The listing builds one solid part. Answer for the finished solid, in the listing's coordinates (mm). A direction names the side the tool comes from. Give positions to 0.01 mm unless a question says otherwise; leave off trailing zeros. Loops run counter-clockwise (first coordinate to the right, second up) from the corner with the lowest first, then second, coordinate; pieces in that order, holes last. Notation, with made-up numbers: (12.25, -32) - (29.25, -32) arc R29 cw to (29.25, -3) - close; hole circle Ø1 at (53.5, -16). An arc over 180 degrees is marked (long way). Write each question's results on one line, items separated by ' | '.
from build123d import *

# Parameters (mm, degrees)
F0_W      = 609.6
F0_H      = 609.6
F0_W_2    = 571.5
F0_H_2    = 571.5
F1_DEPTH  = 381
F3_DEPTH  = 25.4
F5_DEPTH  = 25.4
F6_R      = 5.08
F7_W      = 812.8
F7_H      = 711.2
F8_DEPTH  = 19.05
F9_W      = 812.8
F9_H      = 711.2
F9_W_2    = 774.7
F9_H_2    = 673.1
F10_DEPTH = 101.6
F11_W     = 101.6
F11_H     = 50.8
F12_DEPTH = 711.201
F13_W     = 101.6
F13_H     = 50.8
F14_DEPTH = 812.801


with BuildPart() as f1:
    # F0 (on Top) → F1 (new body, symmetric)
    with BuildSketch(Plane.XY):
        Rectangle(F0_W, F0_H)
        Rectangle(F0_W_2, F0_H_2, mode=Mode.SUBTRACT)
    extrude(amount=F1_DEPTH, both=True)

    # F2 (on face) → F3 (cut)
    with BuildSketch(Plane.XZ.offset(304.8)):
        with BuildLine():
            Line((-228.6, -76.2), (-228.6, -381))
            Line((-228.6, -381), (228.6, -381))
            Line((228.6, -381), (228.6, -76.2))
            ThreePointArc((228.6, -76.2), (0, 152.4), (-228.6, -76.2))
        make_face()
    extrude(amount=-F3_DEPTH, mode=Mode.SUBTRACT)

    # F4 (on face) → F5 (cut)
    with BuildSketch(Plane.YZ.offset(304.8)):
        with BuildLine():
            Line((-228.6, -76.2), (-228.6, -381))
            Line((-228.6, -381), (228.6, -381))
            Line((228.6, -381), (228.6, -76.2))
            ThreePointArc((228.6, -76.2), (0, 152.4), (-228.6, -76.2))
        make_face()
    extrude(amount=-F5_DEPTH, mode=Mode.SUBTRACT)

    # F6
    f6_edges = [f1.edges().sort_by_distance(p)[0] for p in [
        (-228.6, -304.8, -228.6),
        (-228.6, -295.275, -381),
        (-228.6, -285.75, -228.6),
        (-228.6, -295.275, -76.2),
        (0, -304.8, 152.4),
        (0, -285.75, 152.4),
        (228.6, -295.275, -76.2),
        (228.6, -304.8, -228.6),
        (228.6, -285.75, -228.6),
        (228.6, -295.275, -381),
    ]]
    fillet(f6_edges, radius=F6_R)

    # F7 (on face) → F8 (join)
    with BuildSketch(Plane.XY.offset(381)):
        with Locations((0, -50.8)):
            Rectangle(F7_W, F7_H)
    extrude(amount=F8_DEPTH)

    # F9 (on face) → F10 (join)
    with BuildSketch(Plane.XY.offset(400.05)):
        with Locations((0, -50.8)):
            Rectangle(F9_W, F9_H)
        with Locations((0, -50.8)):
            Rectangle(F9_W_2, F9_H_2, mode=Mode.SUBTRACT)
    extrude(amount=F10_DEPTH)

    # F11 (on face) → F12 (cut, through all)
    with BuildSketch(Plane.XZ.offset(406.4)):
        with Locations((-228.6, 476.25)):
            Rectangle(F11_W, F11_H)
        with Locations((-2.54, 476.25)):
            Rectangle(F11_W, F11_H)
        with Locations((223.52, 476.25)):
            Rectangle(F11_W, F11_H)
    extrude(amount=-F12_DEPTH, mode=Mode.SUBTRACT)

    # F13 (on face) → F14 (cut, through all)
    with BuildSketch(Plane(origin=(-406.4, 0, 0), x_dir=(0, -1, 0), z_dir=(-1, 0, 0))):
        with Locations((-152.4, 476.25)):
            Rectangle(F13_W, F13_H)
        with Locations((53.34, 476.25)):
            Rectangle(F13_W, F13_H)
        with Locations((259.08, 476.25)):
            Rectangle(F13_W, F13_H)
    extrude(amount=-F14_DEPTH, mode=Mode.SUBTRACT)


solid = f1.part
Item 1: Flat-ended cylindrical pins translate along their axes: P1, Ø3, axis at x = 217.5, y = 71.5, coming from the -Z side; P2, Ø8, axis at y = -66, z = 156, coming from the -X side; P3, Ø12, axis at x = -62, z = 321, coming from the -Y side. Find the tip coordinate at first contact, or state that the pin passes through.
Values found:
P1: stops at z = 381 | P2: stops at x = -304.8 | P3: stops at y = -304.8
Item 2: For a pull along Y with two mould halves and no side action, classify faces 1 (the face through (5.027, -295.337, 152.345)), 2 (the face through (-4, -285.75, 175)), 3 (the face through (-6, 304.8, 54)) as released by +Y, released by -Y, zero draft, split by the parting line, or undercut.
Values found:
face 1: zero draft | face 2: undercut | face 3: released by +Y
Item 3: Find the intervals of material crossed by line 1 along Y through (x, z) = (23, 429); line 2 along Y through (x, z) = (297, -116); line 3 along Z through (x, y) = (277.5, -141), in increasing order. Write a range as [from, to].
Values found:
line 1: y = [-406.4, -387.35], [285.75, 304.8] | line 2: y = [-304.8, -228.6], [228.6, 304.8] | line 3: z = [381, 400.05]
Item 4: A cutting plane is placed at B-B, the plane x = -258. Determine the outline of the cut face in (y, z).
Values found:
outline: (-406.4, 381) - (-304.8, 381) - (-304.8, -381) - (-285.75, -381) - (-285.75, 381) - (285.75, 381) - (285.75, -381) - (304.8, -381) - (304.8, 450.85) - (285.75, 450.85) - (285.75, 400.05) - (-387.35, 400.05) - (-387.35, 450.85) - (-406.4, 450.85) - close
Item 5: A cutting plane is placed at A-A, the plane z = -269.5. Determine the outline of the cut face in (x, y).
Values found:
outline: (-304.8, -304.8) - (-233.68, -304.8) arc R5.08 ccw to (-228.6, -299.72) - (-228.6, -290.83) arc R5.08 ccw to (-233.68, -285.75) - (-285.75, -285.75) - (-285.75, 285.75) - (285.75, 285.75) - (285.75, 228.6) - (304.8, 228.6) - (304.8, 304.8) - (-304.8, 304.8) - close; (228.6, -299.72) arc R5.08 ccw to (233.68, -304.8) - (304.8, -304.8) - (304.8, -228.6) - (285.75, -228.6) - (285.75, -285.75) - (233.68, -285.75) arc R5.08 ccw to (228.6, -290.83) - close
Item 6: For faces 4 (the face through (285.75, -4, 175)), 5 (the face through (-5, -46, 400.05)), 6 (the face through (295.408, 5.027, 152.345)), determine the directions among +Z, -Z, +X, -X, +Y, -Y from which every point of the face is accessible in a straight line to the end or side of a thin tool.
Values found:
face 4: -Z | face 5: +Z | face 6: -Z, +X
Item 7: A cutting plane is placed at C-C, the plane z = 220.5. Determine the outline of the cut face in (x, y).
Values found:
outline: (-304.8, -304.8) - (304.8, -304.8) - (304.8, 304.8) - (-304.8, 304.8) - close; hole (-285.75, -285.75) - (285.75, -285.75) - (285.75, 285.75) - (-285.75, 285.75) - close
Item 8: A cutting plane is placed at D-D, the plane y = 40.5. Determine the outline of the cut face in (x, z), plus the area to 3 significant figures.
Values found:
outline: (-406.4, 381) - (-304.8, 381) - (-304.8, -381) - (-285.75, -381) - (-285.75, 381) - (285.75, 381) - (285.75, 148.78) - (304.8, 148.78) - (304.8, 381) - (406.4, 381) - (406.4, 501.65) - (387.35, 501.65) - (387.35, 400.05) - (-387.35, 400.05) - (-387.35, 501.65) - (-406.4, 501.65) - close | area: 38,300 mm²
